CAD build for the part. Positions are in the model's coordinates, mm. Coordinates: 2 decimals unless noted, no trailing zeros. Loops run counter-clockwise (first coordinate to the right, second up) from the corner with the lowest first, then second, coordinate; pieces in that order, holes last.
1) Wall check: line 1 along X through (y, z) = (-86.5, 6.75). Give the ranges that are in metal, low to high.
2) Pin check, flat tips, straight feed: pin 1 Ø8 at (x, z) = (11.5, 9.5) entering from +Y; pin 2 Ø3.5 at (y, z) = (-250, 5.5) entering from -X; pin 3 Ø2 at (x, y) = (5, -216.5) entering from -Z. Stop position of each tip, or through.
3) Saw through at B-B, the plane y = -81.5. Write the cut outline in (x, z), and give its area (3 significant figures).
4) Saw through at A-A, the plane z = 6. Write the cut outline in (x, y).
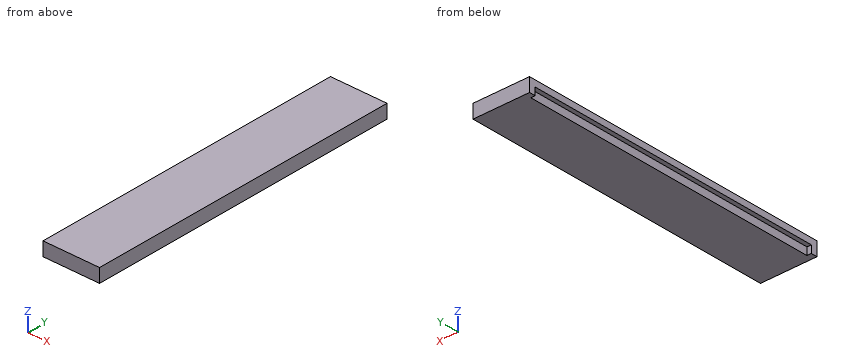
```python
from build123d import *

# Parameters (mm, degrees)
ESQUISSE1_W             = 90.5
ESQUISSE1_H             = 506
BOSS_EXTRU_1_DEPTH      = 22
ESQUISSE2_W             = 12
ESQUISSE2_H             = 486
ENL_V_MAT_EXTRU_1_DEPTH = 7


with BuildPart() as part:
    # Esquisse1 → Boss.-Extru.1 (new body)
    with BuildSketch(Plane.XY):
        with Locations((45.25, -253)):
            Rectangle(ESQUISSE1_W, ESQUISSE1_H)
    extrude(amount=BOSS_EXTRU_1_DEPTH)

    # Esquisse2 → Enlèv. mat.-Extru.1 (cut)
    with BuildSketch(Plane.ZY):
        with Locations((6, -253)):
            Rectangle(ESQUISSE2_W, ESQUISSE2_H)
    extrude(amount=-ENL_V_MAT_EXTRU_1_DEPTH, mode=Mode.SUBTRACT)


solid = part.part
```
Data:
1. line 1: x = 7 to 90.5
2. pin 1: stops at y = 0
2. pin 2: stops at x = 7
2. pin 3: stops at z = 12
3. outline: (0, 12) - (7, 12) - (7, 0) - (90.5, 0) - (90.5, 22) - (0, 22) - close
3. area: 1,910 mm2
4. outline: (0, -506) - (90.5, -506) - (90.5, 0) - (0, 0) - (0, -10) - (7, -10) - (7, -496) - (0, -496) - close
